from build123d import *

# Parameters (mm, degrees)
BOSS_EXTRUDE1_DEPTH = 50.25
CUT_EXTRUDE2_DEPTH  = 3.4
CUT_EXTRUDE2_TAPER  = -5
CHAMFER1_SIZE       = 0.2


with BuildPart() as part:
    # Retainer Profile → Boss-Extrude1 (new body, symmetric)
    with BuildSketch(Plane(origin=(0, 0, 0), x_dir=(0, 0, -1), z_dir=(1, 0, 0))):
        Polygon((-5.1, 4.592304845), (-5.9, 4.592304845), (-5.9, 4.275147558), (-4.5, 2.875147558), (-4.5, 2.192304845), (4.5, 2.192304845), (4.5, 2.875147558), (5.9, 4.275147558), (5.9, 4.592304845), (5.1, 4.592304845), (3, 4.592304845), (3, 3.142304845), (-3, 3.142304845), (-3, 4.592304845), align=None)
    extrude(amount=BOSS_EXTRUDE1_DEPTH, both=True)

    # Sketch3 → Cut-Extrude2 (cut, through all)
    with BuildSketch(Plane(origin=(0, 4.592304845, 0), x_dir=(1, 0, 0), z_dir=(0, 1, 0))):
        Polygon((35.25, 0), (34, 2.165063509), (31.5, 2.165063509), (30.25, 0), (31.5, -2.165063509), (34, -2.165063509), align=None)
        Polygon((2.25, 0), (1, 2.165063509), (-1.5, 2.165063509), (-2.75, 0), (-1.5, -2.165063509), (1, -2.165063509), align=None)
        Polygon((-30.75, 0), (-32, 2.165063509), (-34.5, 2.165063509), (-35.75, 0), (-34.5, -2.165063509), (-32, -2.165063509), align=None)
    extrude(amount=-CUT_EXTRUDE2_DEPTH, taper=CUT_EXTRUDE2_TAPER, mode=Mode.SUBTRACT)

    # Chamfer1
    chamfer1_edges = [part.edges().sort_by_distance(p)[0] for p in [
        (0, 4.592304845, 3),
        (0, 4.592304845, -3),
    ]]
    chamfer(chamfer1_edges, length=CHAMFER1_SIZE)


solid = part.part
For this review, take the finished solid that the model builds, in its own axes (mm). Give positions to 0.01 mm unless a question says otherwise; leave off trailing zeros. Order: outer loops, then holes, each group sorted by start corner. A loop starts at its lowest first (then second) coordinate and runs counter-clockwise, first axis right, second up. Notation, with made-up numbers: (-14, 60) -> (7, 60) arc R10 ccw to (7, 66) -> close; hole circle Ø8 at (-22, 53.25). An arc over 180 degrees is marked (long way). Write item = value, one per line.
1) Insertion check: pin 1 (1 mm diameter, centred on x = 5, y = 3.5, fed in from -Z). The pin has a flat end and moves straight along its axis. Give the tip position at first contact, or say it passes through.
Findings:
pin_1 = -5.62
2) We need section B-B, the plane y = 3.75. Give the boundary of the cut face in (x, z).
Findings:
outline = (-50.25, -5.37) -> (50.25, -5.37) -> (50.25, -3) -> (-50.25, -3) -> close; (-50.25, 3) -> (50.25, 3) -> (50.25, 5.37) -> (-50.25, 5.37) -> close
3) We need section C-C, the plane z = -1.25. Count the separate pieces of the cut face and the enclosed holes in it, and give its area (3 significant figures).
Findings:
separate_pieces = 4
enclosed_holes = 0
area = 84.2 mm^2
4) We need section A-A, the plane x = -14.5. Give the boundary of the cut face in (y, z), and give its area (3 significant figures).
Findings:
outline = (2.19, -4.5) -> (2.88, -4.5) -> (4.28, -5.9) -> (4.59, -5.9) -> (4.59, -3.2) -> (4.39, -3) -> (3.14, -3) -> (3.14, 3) -> (4.39, 3) -> (4.59, 3.2) -> (4.59, 5.9) -> (4.28, 5.9) -> (2.88, 4.5) -> (2.19, 4.5) -> close
area = 15.7 mm^2
5) Draft analysis for pull direction Z (two halves, no side actions). For faces 1 (the face through (1, 4.592, 5)), 2 (the face through (0.7, 3.142, 2.6)), state which applies: pulls with the +Z half, pulls with the -Z half, needs draft (parallel to the pull), parting line crosses it, or undercut.
Findings:
face_1 = needs draft
face_2 = undercut
6) To check wall thickness, follow L1, parallel to X at y = 2.9, z = 2.25; L2, parallel to Z at x = -31.5, y = 3.55; L3, parallel to Z at x = -0.5, y = 2.7. State the ranges of each line that lie inside material, in increasing order. Write a range as from..to.
Findings:
L1 = -50.25..-34.62, -31.88..-1.62, 1.12..31.38, 34.12..50.25
L2 = -5.17..-3, 3..5.17
L3 = -4.5..-2.33, 2.33..4.5
